Answer from the drawing. Dimensions are ordinates in mm from the lowest x, y and z of the part. A direction names the side the tool comes from. Give positions to 0.01 mm unless a question says otherwise; leave off trailing zeros. Loops run counter-clockwise (first coordinate to the right, second up) from the corner with the lowest first, then second, coordinate; pieces in that order, holes last. Notation, with made-up numbers: (-12, -1) - (3, -1) arc R27 ccw to (3, 38) - close; hole circle Ø5 at (-38, 29.25). An arc over 180 degrees is marked (long way). One line per item, written item: value.
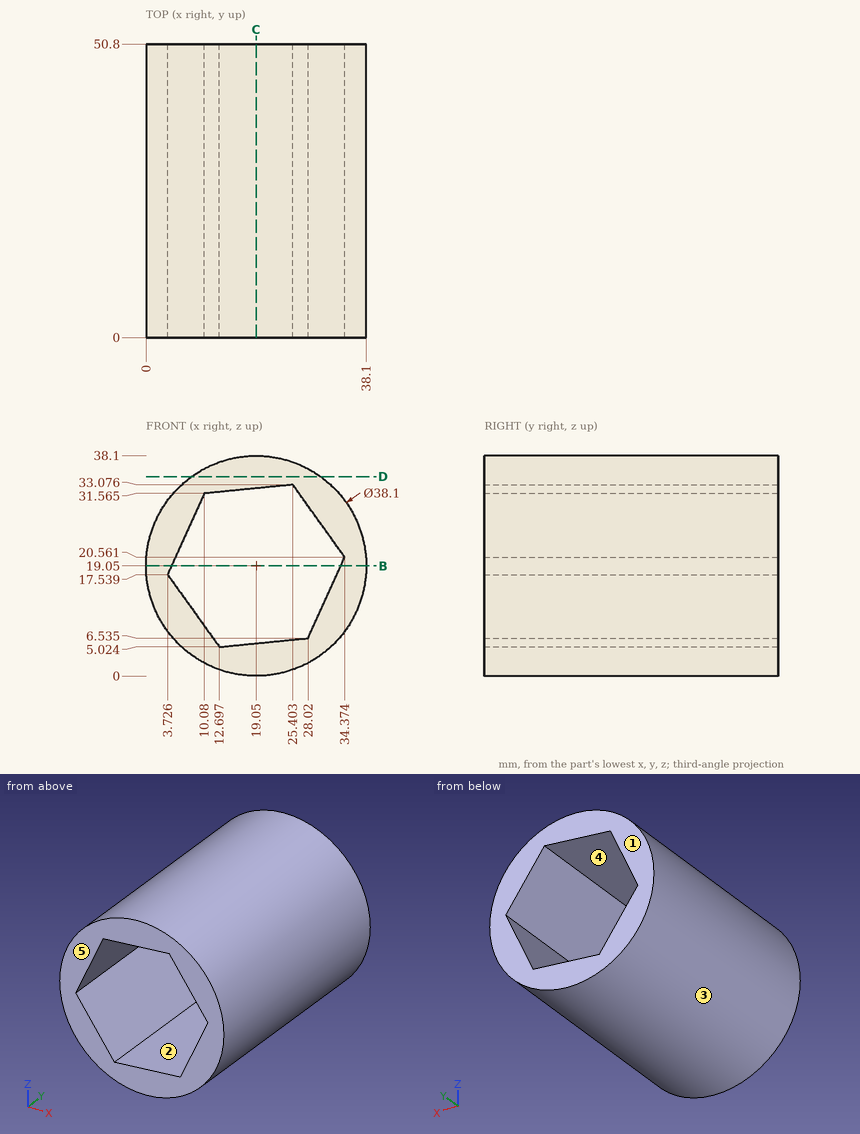
1. For the marked faces 4 and 5, determine the directions among +Z, -Z, +X, -X, +Y, -Y from which every point of the face is accessible in a straight line to the end or side of a thin tool.
Output:
face 4: +Y, -Y
face 5: +Z, -Z, +X, -X, -Y
2. Find the intervals of material crossed by line 1 along X through (y, z) = (38, 18.5); line 2 along X through (y, z) = (28.5, 25) (1 decimal); line 3 along Z through (x, y) = (31, 32) (1 decimal), in increasing order.
Output:
line 1: x = 0.01 to 4.16, 33.44 to 38.09
line 2: x = 1 to 7.1, 31.2 to 37.1
line 3: z = 4.2 to 13.1, 25.3 to 33.9
3. Flat-ended cylindrical pins translate along their axes: pin 1 Ø10 at (x, y) = (23.5, 19.5) entering from -Z; pin 2 Ø3 at (y, z) = (35, 11) entering from -X; pin 3 Ø2 at (x, y) = (19.5, 22.5) entering from +Z. Find the tip coordinate at first contact, or state that the pin passes through.
Output:
pin 1: stops at z = 0
pin 2: stops at x = 1.16
pin 3: stops at z = 38.1
4. The mould has two halves that part along Z. Classify the marked faces 1, 2 and 3: released by +Z, released by -Z, zero draft, split by the parting line, or undercut.
Output:
face 1: zero draft
face 2: undercut
face 3: split by the parting line
5. Section B-B (z = 19.05) is taken. Write down the section's boundary in (x, y).
Output:
outline: (0, 0) - (4.41, 0) - (4.41, 50.8) - (0, 50.8) - close; (33.69, 0) - (38.1, 0) - (38.1, 50.8) - (33.69, 50.8) - close
6. Section D-D (z = 34.5) is taken. Write down the section's boundary in (x, y) (1 decimal).
Output:
outline: (7.9, 0) - (30.2, 0) - (30.2, 50.8) - (7.9, 50.8) - close
7. Section C-C (x = 19.05) is taken. Write down the section's boundary in (y, z), and give its area (3 significant figures).
Output:
outline: (0, 0) - (50.8, 0) - (50.8, 5.65) - (0, 5.65) - close; (0, 32.45) - (50.8, 32.45) - (50.8, 38.1) - (0, 38.1) - close
area: 574 mm²
